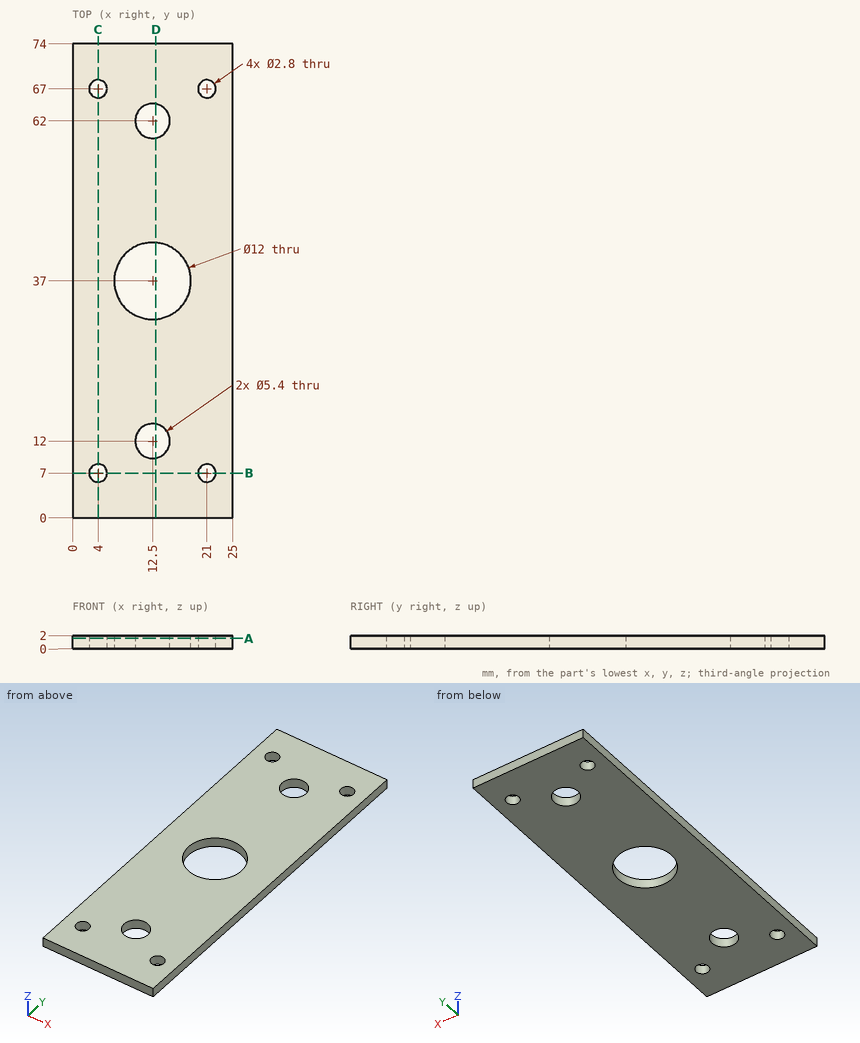
Here's the drawing with two shaded views (mm, measured from the low corner). I have some questions. Coordinates: 2 decimals unless noted, no trailing zeros. Order: outer loops, then holes, each group sorted by start corner. A loop starts at its lowest first (then second) coordinate and runs counter-clockwise, first axis right, second up. Notation, with made-up numbers: (31.5, 9) - (35.5, 9) arc R25 ccw to (35.5, 40) - close; hole circle Ø7 at (74, -7). An arc over 180 degrees is marked (long way). Use CSV: the item, a comma, the result in double quotes. Start each with the question number.
1. Suppose I cut it at B-B on y = 7. List the corners of the cut face in (x, z) for me, then the cut area to 3 significant figures.
2. Suppose I cut it at A-A on z = 1.6. List the corners of the cut face in (x, y) for me.
3. Suppose I cut it at D-D on x = 13. List the corners of the cut face in (y, z) for me, then the cut area to 3 significant figures.
4. Suppose I cut it at C-C on x = 4. List the corners of the cut face in (y, z) for me.
5. Please list where these lines run through material, in increasing order: line 1 (Y direction, x = 12.5, z = 1.1); line 2 (Y direction, x = 4, z = 0.5); line 3 (X direction, y = 67, z = 0.8). Write a range as from..to.
6. I'm going to push a flat-ended pin straight in: pin 1 (3 mm diameter, centred on x = 12.5, y = 62, fed in from +Z). Where does the tip first touch, or does it pass through?
Output:
1,outline,"(0, 0) - (2.6, 0) - (2.6, 2) - (0, 2) - close; (5.4, 0) - (19.6, 0) - (19.6, 2) - (5.4, 2) - close; (22.4, 0) - (25, 0) - (25, 2) - (22.4, 2) - close"
1,area,"38.8 mm2"
2,outline,"(0, 0) - (25, 0) - (25, 74) - (0, 74) - close; hole circle Ø2.8 at (4, 7); hole circle Ø2.8 at (4, 67); hole circle Ø12 at (12.5, 37); hole circle Ø5.4 at (12.5, 12); hole circle Ø5.4 at (12.5, 62); hole circle Ø2.8 at (21, 7); hole circle Ø2.8 at (21, 67)"
3,outline,"(0, 0) - (9.35, 0) - (9.35, 2) - (0, 2) - close; (14.65, 0) - (31.02, 0) - (31.02, 2) - (14.65, 2) - close; (42.98, 0) - (59.35, 0) - (59.35, 2) - (42.98, 2) - close; (64.65, 0) - (74, 0) - (74, 2) - (64.65, 2) - close"
3,area,"103 mm2"
4,outline,"(0, 0) - (5.6, 0) - (5.6, 2) - (0, 2) - close; (8.4, 0) - (65.6, 0) - (65.6, 2) - (8.4, 2) - close; (68.4, 0) - (74, 0) - (74, 2) - (68.4, 2) - close"
5,line 1,"y = 0..9.3, 14.7..31, 43..59.3, 64.7..74"
5,line 2,"y = 0..5.6, 8.4..65.6, 68.4..74"
5,line 3,"x = 0..2.6, 5.4..19.6, 22.4..25"
6,pin 1,"passes through"
